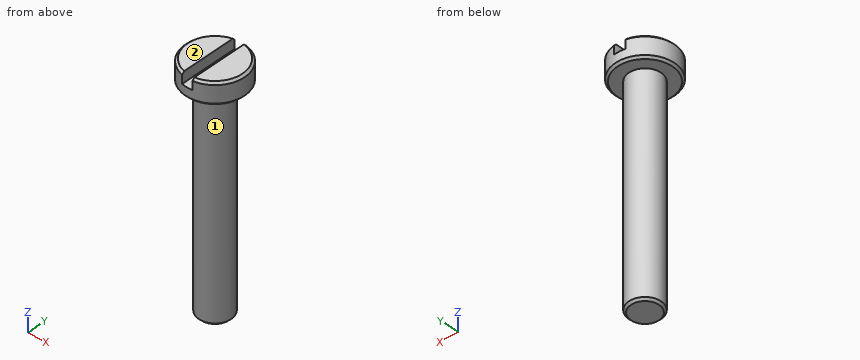
Autodesk Inventor part; units mm, degrees
ref_plane "YZ Plane" through (0, 0, 0) normal (1, 0, 0) x (0, 1, 0)
ref_plane "XZ Plane" through (0, 0, 0) normal (0, 1, 0) x (-1, 0, 0)
ref_plane "XY Plane" through (0, 0, 0) normal (0, 0, 1) x (1, 0, 0)
sketch "Náčrt1" plane through (0, 0, 0) normal (0, 0, 1) x (1, 0, 0)
  circle A0 centre (0, 0) radius 2.75
  dimension "d0" = 5.5
extrude "Vysunutí1" add sketch "Náčrt1" along normal blind 2
chamfer "Zkosení1" distance 0.2 angle 45 1 edges at (-2.75, 0, 2)
chamfer "Zkosení2" distance 0.2 angle 45 1 edges at (-2.75, 0, 0)
sketch "Náčrt2" plane through (0, 0, 2) normal (0, 0, 1) x (1, 0, 0)
  line L0 (-0.6097, -6) -> (0.3903, -6)
  line L1 (0.3903, -6) -> (0.3903, 6)
  line L2 (0.3903, 6) -> (-0.6097, 6)
  line L3 (-0.6097, 6) -> (-0.6097, -6)
  line L4 (-0.6097, -6) -> (0.3903, 6) construction
  line L5 (0.3903, -6) -> (-0.6097, 6) construction
  point P0 (0, 0)
  point P1 (-0.1097, 0)
  dimension "d9" = 1
extrude "Vysunutí2" cut sketch "Náčrt2" against normal blind 1
sketch "Náčrt3" plane through (0, 0, 0) normal (0, 0, -1) x (-1, 0, 0)
  circle A0 centre (0, 0) radius 1.5
  dimension "d12" = 3
extrude "Vysunutí3" add sketch "Náčrt3" along normal blind 20
chamfer "Zkosení3" distance 0.2 angle 45 1 edges at (1.5, 0, -20)
thread "Závit1"
properties part number "Bolt-M3x20" material "Ocel, vysokopevnostní, nízkolegovaná"
The listing builds one solid part. Answer for the finished solid, in the listing's coordinates (mm). Face numbers are marked on the shaded views. A direction names the side the tool comes from. Round coordinates to 2 decimals unless told otherwise and drop trailing zeros. Loops run counter-clockwise (first coordinate to the right, second up) from the corner with the lowest first, then second, coordinate; pieces in that order, holes last. Notation, with made-up numbers: (-9, 72) - (-3, 72) arc R7 cw to (-3, 77) - close; hole circle Ø5 at (6.5, 69.25). An arc over 180 degrees is marked (long way). Return JSON: item names as keys, results as strings. Group by question number.
1. Each of these flat-tipped pins is pushed along its axis until it touches: P1, Ø0.8, axis at y = -0.5, z = 1.5, coming from the +X side; P2, Ø1.5, axis at y = -0.5, z = -5.5, coming from the +X side; P3, Ø3, axis at y = -2, z = -3.5, coming from the +X side. Where does it stop, or does it pass through?
2. Which of the six approach directions +Z, -Z, +X, -X, +Y, -Y give full straight-line access (tool end or side, diameter ignored) to the marked faces 1 and 2?
3. Consider probe 1 along Y at (x, z) = (-0.35, 0.75); probe 2 along X at (y, z) = (-0.75, -13); probe 3 along X at (y, z) = (-0.15, 0.75). Determine where each line is inside the solid, lowest interval first.
4. The part is cut by section B-B on y = 0. Determine the outline of the cut face in (x, z), then the cut area to 3 significant figures.
5. The part is cut by section C-C on z = -13. Determine the outline of the cut face in (x, y).
6. The part is cut by section A-A on x = 0. Determine the outline of the cut face in (y, z).
Resolved:
{
 "1": {"P1": "stops at x = 2.75", "P2": "stops at x = 1.5", "P3": "stops at x = 1.41"},
 "2": {"face 1": "-Z", "face 2": "+Z, +X, -X, +Y, -Y"},
 "3": {"probe 1": "y = -2.73 to 2.73", "probe 2": "x = -1.3 to 1.3", "probe 3": "x = -2.75 to 2.75"},
 "4": {"outline": "(-2.75, 0.2) - (-2.55, 0) - (-1.5, 0) - (-1.5, -19.8) - (-1.3, -20) - (1.3, -20) - (1.5, -19.8) - (1.5, 0) - (2.55, 0) - (2.75, 0.2) - (2.75, 1.8) - (2.55, 2) - (0.39, 2) - (0.39, 1) - (-0.61, 1) - (-0.61, 2) - (-2.55, 2) - (-2.75, 1.8) - close", "area": "69.9 mm²"},
 "5": {"outline": "circle Ø3 at (0, 0)"},
 "6": {"outline": "(-2.75, 0.2) - (-2.55, 0) - (-1.5, 0) - (-1.5, -19.8) - (-1.3, -20) - (1.3, -20) - (1.5, -19.8) - (1.5, 0) - (2.55, 0) - (2.75, 0.2) - (2.75, 1) - (-2.75, 1) - close"}
}
